```python
from build123d import *

# Parameters (mm, degrees)
BASE_FLANGE1_DEPTH          = 1103.3125
SKETCH29_W                  = 76.2
SKETCH29_H                  = 76.2
CUT_EXTRUDE1_DEPTH          = 25.4
F_1_4_CLEARANCE_HOLE5_D     = 6.7564
F_1_4_CLEARANCE_HOLE2_D     = 7.14248
F_1_4_CLEARANCE_HOLE3_D     = 7.14248
F_1_4_CLEARANCE_HOLE4_D     = 6.7564
F_1_2_START                 = -50.8
F_1_2_CLEARANCE_SLOT1_DEPTH = 3.175
SKETCH53_W                  = 50.8
SKETCH53_H                  = 12.7
CUT_EXTRUDE2_DEPTH          = 1112.759017349
TOP_FLANGE_FILLET_R         = 6.35
INTERIOR_CUT_FILLET_R       = 6.35
BOTTOM_EDGE_FILLET_R        = 6.35
SKETCH54_W                  = 12.7
SKETCH54_H                  = 4.7625
CUT_EXTRUDE3_DEPTH          = 1112.759017349
FILLET1_R                   = 0.79375
FILLET2_R                   = 1.5875


# Read off the part's stored shape, not the designer's step: 1/2 Clearance Slot1
# Sheet-metal steps are written as plain solids
with BuildPart() as part:
    # Sketch1 → Base-Flange1 (new body)
    with BuildSketch(Plane(origin=(0, 0, 0), x_dir=(1, 0, 0), z_dir=(0, 1, 0))):
        with BuildLine():
            Line((0, 0), (0, 44.45))
            ThreePointArc((0, 44.45), (1.859871939, 48.940128061), (6.35, 50.8))
            Line((6.35, 50.8), (120.65, 50.8))
            ThreePointArc((120.65, 50.8), (125.140128061, 48.940128061), (127, 44.45))
            Line((127, 44.45), (127, 0))
            Line((127, 0), (123.825, 0))
            Line((123.825, 0), (123.825, 44.45))
            ThreePointArc((123.825, 44.45), (122.89506403, 46.69506403), (120.65, 47.625))
            Line((120.65, 47.625), (6.35, 47.625))
            ThreePointArc((6.35, 47.625), (4.10493597, 46.69506403), (3.175, 44.45))
            Line((3.175, 44.45), (3.175, 0))
            Line((3.175, 0), (0, 0))
        make_face()
    extrude(amount=BASE_FLANGE1_DEPTH)

    # Sketch29 → Cut-Extrude1 (cut)
    with BuildSketch(Plane(origin=(0, 0, -50.8), x_dir=(-1, 0, 0), z_dir=(0, 0, -1))):
        with Locations((-63.5, 862.0125)):
            Rectangle(SKETCH29_W, SKETCH29_H)
    extrude(amount=-CUT_EXTRUDE1_DEPTH, mode=Mode.SUBTRACT)

    # 1/4 Clearance Hole5 (through all)
    with Locations(Plane(origin=(0, 0, -50.8), x_dir=(-1, 0, 0), z_dir=(0, 0, -1))):
        with Locations((-104.775, 53.61305), (-104.775, 288.56305), (-22.225, 288.56305), (-22.225, 53.61305)):
            Hole(F_1_4_CLEARANCE_HOLE5_D / 2)

    # 1/4 Clearance Hole2 (through all)
    with Locations(Plane(origin=(127, 0, 0), x_dir=(0, 0, -1), z_dir=(1, 0, 0))):
        with Locations((19.05, 1074.7375), (19.05, 915.9875)):
            Hole(F_1_4_CLEARANCE_HOLE2_D / 2)

    # 1/4 Clearance Hole3 (through all)
    with Locations(Plane(origin=(0, 0, -50.8), x_dir=(-1, 0, 0), z_dir=(0, 0, -1))):
        with Locations((-107.95, 1074.7375), (-19.05, 1074.7375), (-19.05, 915.9875), (-107.95, 915.9875)):
            Hole(F_1_4_CLEARANCE_HOLE3_D / 2)

    # 1/4 Clearance Hole4 (through all)
    with Locations(Plane(origin=(127, 0, 0), x_dir=(0, 0, -1), z_dir=(1, 0, 0))):
        with Locations((19.05, 221.45625), (19.05, 881.85625)):
            Hole(F_1_4_CLEARANCE_HOLE4_D / 2)

    # 1/2 Clearance Slot1 outline → 1/2 Clearance Slot1 (cut)
    with BuildSketch(Plane.XY.offset(F_1_2_START)):
        with BuildLine():
            Line((71.834375, 619.125), (71.834375, 635))
            ThreePointArc((71.834375, 635), (63.5, 643.334375), (55.165625, 635))
            Line((55.165625, 635), (55.165625, 619.125))
            ThreePointArc((55.165625, 619.125), (63.5, 610.790625), (71.834375, 619.125))
        make_face()
        with BuildLine():
            Line((71.834375, 688.975), (71.834375, 704.85))
            ThreePointArc((71.834375, 704.85), (63.5, 713.184375), (55.165625, 704.85))
            Line((55.165625, 704.85), (55.165625, 688.975))
            ThreePointArc((55.165625, 688.975), (63.5, 680.640625), (71.834375, 688.975))
        make_face()
    extrude(amount=F_1_2_CLEARANCE_SLOT1_DEPTH, mode=Mode.SUBTRACT)

    # Sketch53 → Cut-Extrude2 (cut, through all)
    with BuildSketch(Plane.ZY):
        with Locations((-25.4, 6.35)):
            Rectangle(SKETCH53_W, SKETCH53_H)
    extrude(amount=-CUT_EXTRUDE2_DEPTH, mode=Mode.SUBTRACT)

    # top flange fillet
    top_flange_fillet_edges = [part.edges().sort_by_distance(p)[0] for p in [
        (125.4125, 12.7, 0),
        (1.5875, 12.7, 0),
    ]]
    fillet(top_flange_fillet_edges, radius=TOP_FLANGE_FILLET_R)

    # interior cut fillet
    interior_cut_fillet_edges = [part.edges().sort_by_distance(p)[0] for p in [
        (25.4, 900.1125, -49.2125),
        (25.4, 823.9125, -49.2125),
        (101.6, 823.9125, -49.2125),
        (101.6, 900.1125, -49.2125),
    ]]
    fillet(interior_cut_fillet_edges, radius=INTERIOR_CUT_FILLET_R)

    # bottom edge fillet
    bottom_edge_fillet_edges = [part.edges().sort_by_distance(p)[0] for p in [
        (1.5875, 1103.3125, 0),
        (125.4125, 1103.3125, 0),
    ]]
    fillet(bottom_edge_fillet_edges, radius=BOTTOM_EDGE_FILLET_R)

    # Sketch54 → Cut-Extrude3 (cut, through all)
    with BuildSketch(Plane(origin=(127, 0, 0), x_dir=(0, 0, -1), z_dir=(1, 0, 0))):
        with Locations((6.35, 361.15625)):
            Rectangle(SKETCH54_W, SKETCH54_H)
        Polygon((28.575, 358.06292713), (34.925, 368.3), (31.75, 368.3), (31.75, 384.175), (25.4, 384.175), (25.4, 368.3), (22.225, 368.3), align=None)
    extrude(amount=-CUT_EXTRUDE3_DEPTH, mode=Mode.SUBTRACT)

    # Fillet1
    fillet1_edges = [part.edges().sort_by_distance(p)[0] for p in [
        (125.4125, 358.06292713, -28.575),
        (1.5875, 358.06292713, -28.575),
        (125.4125, 368.3, -22.225),
        (1.5875, 368.3, -22.225),
        (125.4125, 368.3, -25.4),
        (1.5875, 368.3, -25.4),
        (125.4125, 384.175, -25.4),
        (1.5875, 384.175, -25.4),
        (125.4125, 384.175, -31.75),
        (1.5875, 384.175, -31.75),
        (125.4125, 368.3, -31.75),
        (1.5875, 368.3, -31.75),
        (125.4125, 368.3, -34.925),
        (1.5875, 368.3, -34.925),
    ]]
    fillet(fillet1_edges, radius=FILLET1_R)

    # Fillet2
    fillet2_edges = [part.edges().sort_by_distance(p)[0] for p in [
        (125.4125, 358.775, 0),
        (1.5875, 358.775, 0),
        (125.4125, 363.5375, 0),
        (1.5875, 363.5375, 0),
        (125.4125, 363.5375, -12.7),
        (1.5875, 363.5375, -12.7),
        (125.4125, 358.775, -12.7),
        (1.5875, 358.775, -12.7),
    ]]
    fillet(fillet2_edges, radius=FILLET2_R)


solid = part.part
```
Work out the finished part from the listing and answer in its coordinate system (mm). A direction names the side the tool comes from. Round coordinates to 2 decimals unless told otherwise and drop trailing zeros. Write each loop counter-clockwise with the first axis right and the second up, starting at its lowest first coordinate (ties: lowest second). Pieces come first, ordered by that corner, then holes. Notation, with made-up numbers: (-7, 88) - (30, 88) arc R10 cw to (30, 101) - close; hole circle Ø11 at (-25, -21.5). An arc over 180 degrees is marked (long way). Return JSON: item names as keys, results as strings. Group by question number.
Q1. The part is cut by section B-B on y = 117. Write down the section's boundary in (x, z) (3 decimals), then the cut area to 3 significant figures.
Q2. Each of these flat-tipped pins is pushed along its axis until it touches: pin 1 Ø6 at (x, y) = (106.5, 427) entering from +Z (3 decimals); pin 2 Ø1.3 at (x, y) = (1.5, 361) entering from +Z; pin 3 Ø2.5 at (y, z) = (626, -48.5) entering from +X; pin 4 Ø3.5 at (x, z) = (126, -6) entering from -Y. Where does it stop, or does it pass through?
Q3. The part is cut by section A-A on x = 82.5. Write down the section's boundary in (y, z) (1 decimal), then the cut area to 3 significant figures.
Q4. Find the intervals of material crossed by L1, parallel to Y at x = 1, z = -19; L2, parallel to X at y = 345, z = -20.5 (3 decimals); L3, parallel to Z at x = 51.5, y = 134 (3 decimals), in increasing order.
Q5. For faces 1 (the flat face through (69, 1103.312, -48)), 2 (the flat face through (3.175, 550, -23)), determine the directions among +Z, -Z, +X, -X, +Y, -Y from which every point of the face is accessible in a straight line to the end or side of a thin tool.
Q6. The mould has two halves that part along X. Classify faces 3 (the flat face through (123.825, 550, -22)), 4 (the flat face through (0, 550, -22)), 5 (the flat face through (64, 550, -47.625)), 6 (the flat face through (63, 12.7, -48)): released by +X, released by -X, zero draft, split by the parting line, or undercut.
Solved:
{
 "1": {"outline": "(0, -44.45) arc R6.35 ccw to (6.35, -50.8) - (120.65, -50.8) arc R6.35 ccw to (127, -44.45) - (127, 0) - (123.825, 0) - (123.825, -44.45) arc R3.175 cw to (120.65, -47.625) - (6.35, -47.625) arc R3.175 cw to (3.175, -44.45) - (3.175, 0) - (0, 0) - close", "area": "693 mm²"},
 "2": {"pin 1": "z = -47.625", "pin 2": "z = -12.7", "pin 3": "x = 126.35", "pin 4": "y = 12.7"},
 "3": {"outline": "(12.7, -50.8) - (823.9, -50.8) - (823.9, -47.6) - (12.7, -47.6) - close; (900.1, -50.8) - (1103.3, -50.8) - (1103.3, -47.6) - (900.1, -47.6) - close", "area": "3,220 mm²"},
 "4": {"L1": "12.7 to 218.08, 224.83 to 878.48, 885.23 to 912.42, 919.56 to 1071.17, 1078.31 to 1103.31", "L2": "0 to 3.175, 123.825 to 127", "L3": "-50.8 to -47.625"},
 "5": {"face 1": "+Z, -Z, +X, -X, +Y", "face 2": "+Z, +Y, -Y"},
 "6": {"face 3": "undercut", "face 4": "released by -X", "face 5": "undercut", "face 6": "zero draft"}
}
